```python
from build123d import *

# Parameters (mm, degrees)
BOSS_EXTRUDE1_DEPTH = 16
FILLET1_R           = 10
SKETCH2_R           = 4
CUT_EXTRUDE1_DEPTH  = 16
SKETCH3_R           = 2
CUT_EXTRUDE2_DEPTH  = 24


with BuildPart() as part:
    # Sketch1 → Boss-Extrude1 (new body)
    with BuildSketch(Plane(origin=(0, 0, 0), x_dir=(1, 0, 0), z_dir=(0, 1, 0))):
        Polygon((-11, 20), (-11, -20), (-6.5, -20), (-6.5, 8), (6.5, 8), (6.5, -20), (11, -20), (11, 20), align=None)
    extrude(amount=BOSS_EXTRUDE1_DEPTH)

    # Fillet1
    fillet1_edges = [part.edges().sort_by_distance(p)[0] for p in [
        (-8.75, 16, 20),
        (8.75, 16, 20),
    ]]
    fillet(fillet1_edges, radius=FILLET1_R)

    # Sketch2 → Cut-Extrude1 (cut)
    with BuildSketch(Plane(origin=(0, 0, -20), x_dir=(-1, 0, 0), z_dir=(0, 0, -1))):
        with Locations((0, 7.920875605)):
            Circle(SKETCH2_R)
    extrude(amount=-CUT_EXTRUDE1_DEPTH, mode=Mode.SUBTRACT)

    # Sketch3 → Cut-Extrude2 (cut)
    with BuildSketch(Plane.ZY.offset(11)):
        with Locations((12.5, 8)):
            Circle(SKETCH3_R)
    extrude(amount=-CUT_EXTRUDE2_DEPTH, mode=Mode.SUBTRACT)


solid = part.part
```
Geometry check sheet. Reference: the model listing, model coordinates, mm. A direction names the side the tool comes from. Give positions to 0.01 mm unless a question says otherwise; leave off trailing zeros. Order: outer loops, then holes, each group sorted by start corner. A loop starts at its lowest first (then second) coordinate and runs counter-clockwise, first axis right, second up.
1. Release check for a two-part mould opening along X. For faces 1 (the face through (8.78, 12.99, 17.15)), 2 (the face through (-11, 8, 0)), 3 (the face through (0.867, 4.016, -14.084)), 4 (the face through (-4.4, 7.9, -8)) record: pulls with the +X half, pulls with the -X half, needs draft (parallel to the pull), parting line crosses it, or undercut.
2. Section check B-B, the plane x = 0. Enter the section's corners in (y, z), and give its area (3 significant figures).
3. Thickness scan on L1, parallel to X at y = 8.25, z = 17; L2, parallel to Y at x = 0, z = -14.75; L3, parallel to Z at x = -4, y = 2.5. Record the ranges inside material, lowest first.
4. Section check D-D, the plane y = 9. Enter the section's corners in (x, z), and give its area (3 significant figures).
5. Access from +Z, -Z, +X, -X, +Y, -Y to the whole of each face (thin tool, end or side, straight path). Record for faces 5 (the face through (6.5, 8, 6)), 6 (the face through (8.718, 9.352, 11.026)).
6. Section check C-C, the plane y = 5. Enter the section's corners in (x, z).
7. Gauge pin test, flat ends, axial feed: pin 1 Ø3 at (y, z) = (8, 12.5) entering from +X; pin 2 Ø1.5 at (x, y) = (-4.5, 3) entering from +Z; pin 3 Ø4 at (x, z) = (6, -16) entering from -Y. Record the tip position at first contact, or that the pin passes through.
8. Section check A-A, the plane z = -2. Enter the section's corners in (x, y).
Values follow:
1. face 1: needs draft
1. face 2: pulls with the -X half
1. face 3: undercut
1. face 4: undercut
2. outline: (0, -20) - (3.92, -20) - (3.92, -8) - (0, -8) - close; (11.92, -20) - (16, -20) - (16, -8) - (11.92, -8) - close
2. area: 96.0 mm2
3. L1: x = -11 to -6.5, 6.5 to 11
3. L2: y = 0 to 3.92, 11.92 to 16
3. L3: z = -20 to -8
4. outline: (-11, -20) - (-3.85, -20) - (-3.85, -8) - (-6.5, -8) - (-6.5, 10.77) - (-11, 10.77) - close; (-11, 14.23) - (-6.5, 14.23) - (-6.5, 19.54) - (-11, 19.54) - close; (3.85, -20) - (11, -20) - (11, 10.77) - (6.5, 10.77) - (6.5, -8) - (3.85, -8) - close; (6.5, 14.23) - (11, 14.23) - (11, 19.54) - (6.5, 19.54) - close
4. area: 388 mm2
5. face 5: +Z, +Y, -Y
5. face 6: +X, -X
6. outline: (-11, -20) - (-2.73, -20) - (-2.73, -8) - (-6.5, -8) - (-6.5, 20) - (-11, 20) - close; (2.73, -20) - (11, -20) - (11, 20) - (6.5, 20) - (6.5, -8) - (2.73, -8) - close
7. pin 1: passes through
7. pin 2: stops at z = -8
7. pin 3: stops at y = 0
8. outline: (-11, 0) - (-6.5, 0) - (-6.5, 16) - (-11, 16) - close; (6.5, 0) - (11, 0) - (11, 16) - (6.5, 16) - close
